from build123d import *

# Parameters (mm, degrees)
F0_R           = 17.4912065647
F2_DEPTH       = 35.941
F1_W           = 6.9445110857
F1_H           = 61.1279271543
F3_DEPTH       = 17.526
F3_DEPTH_BACK  = 17.526
F1_W_2         = 6.845775526
F4_DEPTH       = 17.526
F4_DEPTH_BACK  = 17.526
F6_DEPTH       = 35.941
F8_DEPTH       = 25.4
F8_DEPTH_BACK  = 25.4
F9_R           = 10.1290533854
F9_R_2         = 10.4269018425
F10_DEPTH      = 38.1
F10_DEPTH_BACK = 38.1


with BuildPart() as f2:
    # F0 (on Front) → F2 (new body)
    with BuildSketch(Plane.XZ):
        Circle(F0_R)
    extrude(amount=-F2_DEPTH)

    # F1 (on Right) → F3 (join, two sides)
    with BuildSketch(Plane.YZ) as f3_sk:
        with Locations((32.4680674821, 30.5639635772)):
            Rectangle(F1_W, F1_H)
    extrude(amount=F3_DEPTH)
    extrude(f3_sk.sketch, amount=-F3_DEPTH_BACK)

    # F1 (on Right) → F4 (join, two sides)
    with BuildSketch(Plane.YZ) as f4_sk:
        with Locations((3.422887763, 30.5639635772)):
            Rectangle(F1_W_2, F1_H)
        with Locations((32.4680674821, 30.5639635772)):
            Rectangle(F1_W, F1_H)
    extrude(amount=F4_DEPTH)
    extrude(f4_sk.sketch, amount=-F4_DEPTH_BACK)

    # F5 (on face) → F6 (join)
    with BuildSketch(Plane.XZ):
        with BuildLine():
            Line((-17.526, 61.1279271543), (17.526, 61.1279271543))
            ThreePointArc((17.526, 61.1279271543), (0, 73.8669370431), (-17.526, 61.1279271543))
        make_face()
    extrude(amount=-F6_DEPTH)

    # F7 (on Right) → F8 (cut, two sides)
    with BuildSketch(Plane.YZ) as f8_sk:
        Polygon((6.9377436303, 74.695661664), (6.9377436303, 60.9454773366), (28.9229359478, 60.8699284494), (28.9229359478, 74.2423608899), align=None)
    extrude(amount=F8_DEPTH, mode=Mode.SUBTRACT)
    extrude(f8_sk.sketch, amount=-F8_DEPTH_BACK, mode=Mode.SUBTRACT)

    # F9 (on face) → F10 (cut, two sides)
    with BuildSketch(Plane.XZ) as f10_sk:
        with Locations((0, 58.616951108)):
            Circle(F9_R)
        Circle(F9_R_2)
    extrude(amount=F10_DEPTH, mode=Mode.SUBTRACT)
    extrude(f10_sk.sketch, amount=-F10_DEPTH_BACK, mode=Mode.SUBTRACT)


solid = f2.part
Design review of the part built by this model. Coordinates are the model's own, in mm. A direction names the side the tool comes from. Round coordinates to 2 decimals unless told otherwise and drop trailing zeros. Write each loop counter-clockwise with the first axis right and the second up, starting at its lowest first coordinate (ties: lowest second). Pieces come first, ordered by that corner, then holes. Notation, with made-up numbers: (37, -33) - (67, -33) arc R17 cw to (67, 0) - close; hole circle Ø4 at (63, -32). An arc over 180 degrees is marked (long way). Return JSON: item names as keys, results as strings. Group by question number.
Item 1: The part is to be moulded in two halves that separate along Z. For faces 1 (the face through (-17.526, 3, 31)), 2 (the face through (-1.32, 3.42, 68.66)), 3 (the face through (-2.26, 17.72, -10.18)), 4 (the face through (0.324, 32.383, 73.864)), say which applies: pulls with the +Z half, pulls with the -Z half, needs draft (parallel to the pull), parting line crosses it, or undercut.
Item 2: We need section C-C on z = 56.5. Write out the cut boundary in (x, y), and give its area (3 significant figures).
Item 3: Machinability: for faces 5 (the face through (8.07, 17.72, -15.52)), 6 (the face through (-17.526, 32, 31)), 7 (the face through (0, 6.938, 69)), which of the approach directions +Z, -Z, +X, -X, +Y, -Y give a long, thin tool a straight path to every point of the face, cutting with its end or side? Answer none if there is none.
Item 4: For probe 1 along Z at (x, y) = (0, 34); probe 2 along Y at (x, z) = (15, 41); probe 3 along Y at (x, z) = (14, 65.5), list the stretches that pass through material, from the lowest coordinate up. Write a range as [from, to].
Item 5: We need section A-A on z = 32. Write out the cut boundary in (x, y).
Item 6: Insertion check: P1, Ø6, axis at y = 32, z = -0.5, coming from the -X side; P2, Ø18, axis at x = 0, z = 58.62, coming from the +Y side; P3, Ø8, axis at x = -8, y = 27, coming from the -Z side; P4, Ø1, axis at x = -13.5, y = 10.5, coming from the +Z side. Each pin has a flat end and moves straight along its axis. Give the tip position at first contact, or say it passes through.
Item 7: We need section B-B on x = 0. Give the number of separate pieces and of enclosed holes in the cut face, and give its area (3 significant figures).
Model answer:
{
 "1": {"face 1": "needs draft", "face 2": "undercut", "face 3": "undercut", "face 4": "pulls with the +Z half"},
 "2": {"outline": "(-17.53, 0) - (-9.91, 0) - (-9.91, 6.85) - (-17.53, 6.85) - close; (-17.53, 29) - (-9.91, 29) - (-9.91, 35.94) - (-17.53, 35.94) - close; (9.91, 0) - (17.53, 0) - (17.53, 6.85) - (9.91, 6.85) - close; (9.91, 29) - (17.53, 29) - (17.53, 35.94) - (9.91, 35.94) - close", "area": "210 mm²"},
 "3": {"face 5": "none", "face 6": "+Z, -Z, -X, +Y, -Y", "face 7": "+Z, +X, -X"},
 "4": {"probe 1": "z = [-17.49, -10.43], [10.43, 48.49], [68.75, 73.87]", "probe 2": "y = [0, 6.85], [29, 35.94]", "probe 3": "y = [0, 6.94], [28.92, 35.94]"},
 "5": {"outline": "(-17.53, 0) - (17.53, 0) - (17.53, 6.85) - (-17.53, 6.85) - close; (-17.53, 29) - (17.53, 29) - (17.53, 35.94) - (-17.53, 35.94) - close"},
 "6": {"P1": "stops at x = -17.53", "P2": "passes through", "P3": "stops at z = -17.03", "P4": "stops at z = 11.7"},
 "7": {"separate pieces": "4", "enclosed holes": "0", "area": "1,010 mm²"}
}
